Work out the finished part from the listing and answer in its coordinate system (mm). Face numbers are marked on the shaded views. A direction names the side the tool comes from. Coordinates: 2 decimals unless noted, no trailing zeros. Loops run counter-clockwise (first coordinate to the right, second up) from the corner with the lowest first, then second, coordinate; pieces in that order, holes last. Notation, with made-up numbers: (34, -10.5) -> (59, -10.5) arc R10 ccw to (59, 5.5) -> close; hole circle Ø11 at (37, -30). An arc over 180 degrees is marked (long way). One line per question, with ' | ' between items.
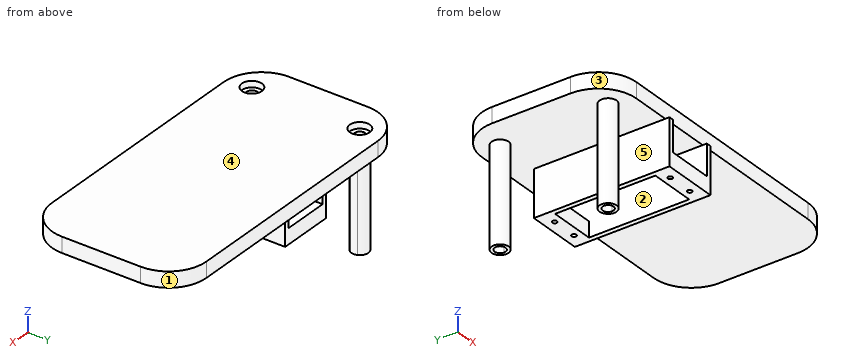
```python
from build123d import *

# Parameters (mm, degrees)
SKETCH1_W              = 180
SKETCH1_H              = 100
BOSS_EXTRUDE1_DEPTH    = 10
FILLET1_R              = 24.5
SKETCH5_R              = 5.5
SKETCH5_R_2            = 3.5
BOSS_EXTRUDE4_DEPTH    = 64
MOVE_FACE2_DEPTH       = 10
MOVE_START             = -64
MOVE_FACE3_OUTLINE_R   = 3.5
MOVE_FACE3_DEPTH       = 64
MOVE_FACE3_2_DEPTH     = 10
MOVE_FACE3_3_OUTLINE_R = 3.5
MOVE_FACE3_3_DEPTH     = 64
SKETCH7_R              = 3.5
CUT_EXTRUDE2_DEPTH     = 74
SKETCH8_R              = 6.5
CUT_EXTRUDE3_DEPTH     = 4
SKETCH9_W              = 36.05660051
SKETCH9_H              = 87.936885764
SKETCH9_R              = 1.5
SKETCH9_W_2            = 29.8
SKETCH9_H_2            = 65
BOSS_EXTRUDE6_DEPTH    = 10
SKETCH10_W             = 3.128300255
SKETCH10_H             = 87.936885764
BOSS_EXTRUDE7_DEPTH    = 20


# Read off the part's stored shape, not the designer's step: Move Face2, Move Face3
with BuildPart() as part:
    # Sketch1 → Boss-Extrude1 (new body)
    with BuildSketch(Plane.XY):
        Rectangle(SKETCH1_W, SKETCH1_H)
    extrude(amount=BOSS_EXTRUDE1_DEPTH)

    # Fillet1
    fillet1_edges = [part.edges().sort_by_distance(p)[0] for p in [
        (90, -50, 5),
        (-90, -50, 5),
        (-90, 50, 5),
        (90, 50, 5),
    ]]
    fillet(fillet1_edges, radius=FILLET1_R)

    # Sketch5 → Boss-Extrude4 (add)
    # profile 1 of 2: a face of its own
    with BuildSketch(Plane(origin=(0, 0, 0), x_dir=(-1, 0, 0), z_dir=(0, 0, -1))):
        with Locations((80, 35)):
            Circle(SKETCH5_R)
        with Locations((80, 35)):
            Circle(SKETCH5_R_2, mode=Mode.SUBTRACT)
    # profile 2 of 2: a face of its own
    with BuildSketch(Plane(origin=(0, 0, 0), x_dir=(-1, 0, 0), z_dir=(0, 0, -1))):
        with Locations((80, -35)):
            Circle(SKETCH5_R)
        with Locations((80, -35)):
            Circle(SKETCH5_R_2, mode=Mode.SUBTRACT)
    extrude(amount=BOSS_EXTRUDE4_DEPTH)

    # Move Face2 outline → Move Face2 (add)
    with BuildSketch(Plane.XY):
        with BuildLine():
            Line((-100, 25.5), (-100, -25.5))
            ThreePointArc((-100, -25.5), (-92.824116139, -42.824116139), (-75.5, -50))
            Line((-75.5, -50), (-65.5, -50))
            ThreePointArc((-65.5, -50), (-82.824116139, -42.824116139), (-90, -25.5))
            Line((-90, -25.5), (-90, 25.5))
            ThreePointArc((-90, 25.5), (-82.824116139, 42.824116139), (-65.5, 50))
            Line((-65.5, 50), (-75.5, 50))
            ThreePointArc((-75.5, 50), (-92.824116139, 42.824116139), (-100, 25.5))
        make_face()
    extrude(amount=MOVE_FACE2_DEPTH)

    # Move Face3 outline → Move Face3 (cut)
    # profile 1 of 2: a face of its own
    with BuildSketch(Plane.XY.offset(MOVE_START)):
        with BuildLine():
            ThreePointArc((-85, 37.291287847), (-84.5, 35), (-85, 32.708712153))
            ThreePointArc((-85, 32.708712153), (-74.5, 35), (-85, 37.291287847))
        make_face()
        with Locations((-80, 35)):
            Circle(MOVE_FACE3_OUTLINE_R, mode=Mode.SUBTRACT)
    # profile 2 of 2: a face of its own
    with BuildSketch(Plane.XY.offset(MOVE_START)):
        with BuildLine():
            ThreePointArc((-85, -32.708712153), (-84.5, -35), (-85, -37.291287847))
            ThreePointArc((-85, -37.291287847), (-74.5, -35), (-85, -32.708712153))
        make_face()
        with Locations((-80, -35)):
            Circle(MOVE_FACE3_OUTLINE_R, mode=Mode.SUBTRACT)
    extrude(amount=MOVE_FACE3_DEPTH, mode=Mode.SUBTRACT)

    # Move Face3 2 outline → Move Face3 2 (add)
    with BuildSketch(Plane.XY):
        with BuildLine():
            Line((-110, 25.5), (-110, -25.5))
            ThreePointArc((-110, -25.5), (-102.824116139, -42.824116139), (-85.5, -50))
            Line((-85.5, -50), (-75.5, -50))
            ThreePointArc((-75.5, -50), (-92.824116139, -42.824116139), (-100, -25.5))
            Line((-100, -25.5), (-100, 25.5))
            ThreePointArc((-100, 25.5), (-92.824116139, 42.824116139), (-75.5, 50))
            Line((-75.5, 50), (-85.5, 50))
            ThreePointArc((-85.5, 50), (-102.824116139, 42.824116139), (-110, 25.5))
        make_face()
    extrude(amount=MOVE_FACE3_2_DEPTH)

    # Move Face3 3 outline → Move Face3 3 (add)
    # profile 1 of 2: a face of its own
    with BuildSketch(Plane.XY.offset(MOVE_START)):
        with BuildLine():
            ThreePointArc((-85, 32.708712153), (-85.5, 35), (-85, 37.291287847))
            ThreePointArc((-85, 37.291287847), (-95.5, 35), (-85, 32.708712153))
        make_face()
        with Locations((-90, 35)):
            Circle(MOVE_FACE3_3_OUTLINE_R, mode=Mode.SUBTRACT)
    # profile 2 of 2: a face of its own
    with BuildSketch(Plane.XY.offset(MOVE_START)):
        with BuildLine():
            ThreePointArc((-85, -37.291287847), (-85.5, -35), (-85, -32.708712153))
            ThreePointArc((-85, -32.708712153), (-95.5, -35), (-85, -37.291287847))
        make_face()
        with Locations((-90, -35)):
            Circle(MOVE_FACE3_3_OUTLINE_R, mode=Mode.SUBTRACT)
    extrude(amount=MOVE_FACE3_3_DEPTH)

    # Sketch7 → Cut-Extrude2 (cut)
    with BuildSketch(Plane(origin=(0, 0, -64), x_dir=(-1, 0, 0), z_dir=(0, 0, -1))):
        with Locations((90, -35)):
            Circle(SKETCH7_R)
        with Locations((90, 35)):
            Circle(SKETCH7_R)
    extrude(amount=-CUT_EXTRUDE2_DEPTH, mode=Mode.SUBTRACT)

    # Sketch8 → Cut-Extrude3 (cut)
    with BuildSketch(Plane.XY.offset(10)):
        with Locations((-90, 35)):
            Circle(SKETCH8_R)
        with Locations((-90, -35)):
            Circle(SKETCH8_R)
    extrude(amount=-CUT_EXTRUDE3_DEPTH, mode=Mode.SUBTRACT)



with BuildPart() as body_2:
    # Sketch9 → Boss-Extrude6 (new body)
    with BuildSketch(Plane(origin=(0, 0, -30), x_dir=(-1, 0, 0), z_dir=(0, 0, -1))):
        with Locations((42, -8.75)):
            Rectangle(SKETCH9_W, SKETCH9_H)
        with Locations((33.5, 28.75)):
            Circle(SKETCH9_R, mode=Mode.SUBTRACT)
        with Locations((50.5, 28.75)):
            Circle(SKETCH9_R, mode=Mode.SUBTRACT)
        with Locations((50.5, -46.25)):
            Circle(SKETCH9_R, mode=Mode.SUBTRACT)
        with Locations((33.5, -46.25)):
            Circle(SKETCH9_R, mode=Mode.SUBTRACT)
        with Locations((42, -8.75)):
            Rectangle(SKETCH9_W_2, SKETCH9_H_2, mode=Mode.SUBTRACT)
    extrude(amount=-BOSS_EXTRUDE6_DEPTH)


with BuildPart() as part_1:
    add(part.part)

    add(body_2.part)  # Boss-Extrude7 merges body 2
    # Sketch10 → Boss-Extrude7 (add)
    with BuildSketch(Plane.XY.offset(-20)):
        with Locations((-25.535849873, -8.75)):
            Rectangle(SKETCH10_W, SKETCH10_H)
        with Locations((-58.464150128, -8.75)):
            Rectangle(SKETCH10_W, SKETCH10_H)
    extrude(amount=BOSS_EXTRUDE7_DEPTH)


solid = part_1.part
```
1) Find section A-A (z = -7). Write down the section's boundary in (x, y).
Check values:
outline: circle Ø11 at (-90, -35); circle Ø11 at (-90, 35); (-60.03, -52.72) -> (-56.9, -52.72) -> (-56.9, 35.22) -> (-60.03, 35.22) -> close; (-27.1, -52.72) -> (-23.97, -52.72) -> (-23.97, 35.22) -> (-27.1, 35.22) -> close; hole circle Ø7 at (-90, -35); hole circle Ø7 at (-90, 35)
2) Find section D-D (y = 4). Write down the section's boundary in (x, z).
Check values:
outline: (-110, 0) -> (-60.03, 0) -> (-60.03, -30) -> (-56.9, -30) -> (-56.9, 0) -> (-27.1, 0) -> (-27.1, -30) -> (-23.97, -30) -> (-23.97, 0) -> (90, 0) -> (90, 10) -> (-110, 10) -> close
3) Find section C-C (x = -45). Write down the section's boundary in (y, z), plus the area to 3 significant figures.
Check values:
outline: (-52.72, -30) -> (-41.25, -30) -> (-41.25, -20) -> (-52.72, -20) -> close; (-50, 0) -> (50, 0) -> (50, 10) -> (-50, 10) -> close; (23.75, -30) -> (35.22, -30) -> (35.22, -20) -> (23.75, -20) -> close | area: 1,230 mm^2
4) Flat-ended cylindrical pins translate along their axes: pin 1 (1.8 mm diameter, centred on x = -50.5, y = 28.75, fed in from -Z); pin 2 (10 mm diameter, centred on y = 33, z = -52.5, fed in from -X); pin 3 (11 mm diameter, centred on x = -33.5, z = 3.5, fed in from -Y). Find the tip coordinate at first contact, or state that the pin passes through.
Check values:
pin 1: stops at z = 0 | pin 2: stops at x = -95.5 | pin 3: stops at y = -50
5) The mould has two halves that part along X. Classify the marked faces 1, 2 and 3: released by +X, released by -X, zero draft, split by the parting line, or undercut.
Check values:
face 1: released by +X | face 2: undercut | face 3: released by -X
6) Find section B-B (z = -54). Write down the section's boundary in (x, y), plus the area to 3 significant figures.
Check values:
outline: circle Ø11 at (-90, -35); circle Ø11 at (-90, 35); hole circle Ø7 at (-90, -35); hole circle Ø7 at (-90, 35) | area: 113 mm^2
7) Find the intervals of material crossed by line 1 along Y through (x, z) = (-50.5, -23); line 2 along X through (y, z) = (-46, -26); line 3 along X through (y, z) = (34.5, -17.5), in increasing order.
Check values:
line 1: y = -52.72 to -47.75, -44.75 to -41.25, 23.75 to 27.25, 30.25 to 35.22 | line 2: x = -60.03 to -51.98, -49.02 to -34.98, -32.02 to -23.97 | line 3: x = -95.48 to -93.46, -86.54 to -84.52, -60.03 to -56.9, -27.1 to -23.97
8) For the marked faces 4 and 5, determine the directions among +Z, -Z, +X, -X, +Y, -Y from which every point of the face is accessible in a straight line to the end or side of a thin tool.
Check values:
face 4: +Z, +X, -X, +Y, -Y | face 5: -Z, +Y, -Y
